Source: CAD feature listing. Evaluate the final solid. Frame: model axes, mm. A direction names the side the tool comes from. Round coordinates to 2 decimals unless told otherwise and drop trailing zeros. Loops run counter-clockwise (first coordinate to the right, second up) from the corner with the lowest first, then second, coordinate; pieces in that order, holes last. Notation, with made-up numbers: M -2,-27.75 L 26,-27.75 A35 cw 26,8.25 Z; hole C 86.5,7 d10. An arc over 180 degrees is marked long. Write each question's results on one line, items separated by ' | '. Start each with the question number.
1. Draft query along X for faces 1 (the flat face through (3, 14, 7)), 2 (the cylindrical face through (0.6, 27.43, 5.58)), 3 (the flat face through (101, 14, 1)), 4 (the flat face through (63.7, 25.2, 12)). Return one class per face: released by +X, released by -X, zero draft, split by the parting line, or undercut.
2. Ray query, line 1 (Y direction, x = 64, z = 8); line 2 (Y direction, x = 37, z = 9.75); line 3 (Z direction, x = 116, y = 22.25). Return the intervals inside material, ascending.
3. Section B-B on x = 58.5. Output: boundary loops of the cut face in (y, z).
4. Section C-C on x = 117. Output: boundary loops of the cut face in (y, z), and give its area (3 significant figures).
5. Set-up query: faces 5 (the flat face through (0, 14, 5)), 6 (the flat face through (64, 14, 2)), 7 (the flat face through (127, 14, 6)). Return all of +Z, -Z, +X, -X, +Y, -Y with unobstructed straight access to the full face (end or side cutting, diameter ignored); none if empty.
6. Section A-A on z = 9.75. Output: boundary loops of the cut face in (x, y).
7. Contact query for flat-ended pins moving along their axis: pin 1 Ø0.6 at (x, y) = (64.5, 14) entering from +Z; pin 2 Ø0.5 at (x, z) = (54, 11.5) entering from +Y; pin 3 Ø4 at (x, y) = (87.5, 18) entering from +Z. Output: stop coordinate, or through.
Autodesk Inventor part; units mm, degrees
ref_plane "Work Plane7" through (0, 0, 12) normal (0, 0, 1) x (1, 0, 0)
ref_plane "Work Plane6" through (0, 0, 12) normal (0, 0, 1) x (1, 0, 0)
ref_plane "Work Plane5" through (0, 0, 12) normal (0, 0, 1) x (1, 0, 0)
sketch "Sketch1" plane through (0, 0, 0) normal (0, 0, 1) x (1, 0, 0)
  line L0 (0, 0) -> (128, 0)
  line L1 (128, 0) -> (128, 28)
  line L2 (128, 28) -> (0, 28)
  line L3 (0, 28) -> (0, 0)
  dimension "d57" = 128
  dimension "d58" = 28
ref_plane "Work Plane7" through (0, 0, 12) normal (0, 0, 1) x (1, 0, 0)
sketch "Sketch2" plane through (0, 0, 12) normal (0, 0, 1) x (1, 0, 0)
  line L0 (3, 3) -> (85, 3)
  line L1 (85, 3) -> (85, 45)
  line L2 (85, 45) -> (3, 45)
  line L3 (3, 45) -> (3, 3)
  line L4 (88, 48) -> (0, 48)
  line L5 (88, 0) -> (88, 48)
  line L6 (0, 0) -> (88, 0)
  line L7 (0, 48) -> (0, 0)
  dimension "d4" = 3
  dimension "d5" = 3
  dimension "d6" = 3
  dimension "d7" = 3
ref_plane "Work Plane6" through (0, 0, 12) normal (0, 0, 1) x (1, 0, 0)
sketch "Sketch3" plane through (0, 0, 12) normal (0, 0, 1) x (1, 0, 0)
  line L0 (1.5, 46.5) -> (86.5, 46.5)
  line L1 (86.5, 46.5) -> (86.5, 1.5)
  line L2 (86.5, 1.5) -> (1.5, 1.5)
  line L3 (1.5, 1.5) -> (1.5, 46.5)
  line L4 (0, 0) -> (88, 0)
  line L5 (0, 48) -> (0, 0)
  line L6 (88, 0) -> (0, 0)
  line L7 (0, 0) -> (0, 48)
  line L8 (0, 48) -> (88, 48)
  line L9 (88, 48) -> (88, 0)
  dimension "d10" = 1.5
  dimension "d11" = 1.5
  dimension "d12" = 1.5
  dimension "d13" = 1.5
ref_plane "Work Plane5" through (0, 0, 12) normal (0, 0, 1) x (1, 0, 0)
sketch "Sketch4" plane through (0, 0, 12) normal (0, 0, 1) x (1, 0, 0)
  circle A0 centre (5.5, 24) radius 1
  circle A1 centre (82.5, 24) radius 1
  line L0 (3, 45) -> (85, 45)
  line L1 (3, 3) -> (3, 45)
  line L2 (3, 25.5) -> (5.5, 25.5)
  line L3 (5.5, 25.5) -> (5.5, 22.5)
  line L4 (5.5, 22.5) -> (3, 22.5)
  line L5 (3, 22.5) -> (3, 25.5)
  circle A2 centre (5.5, 24) radius 1.5
  line L6 (85, 45) -> (85, 3)
  line L7 (85, 22.5) -> (82.5, 22.5)
  line L8 (82.5, 22.5) -> (82.5, 25.5)
  line L9 (82.5, 25.5) -> (85, 25.5)
  line L10 (85, 25.5) -> (85, 22.5)
  circle A3 centre (82.5, 24) radius 1.5
  point P0 (0, 0)
  dimension "d17" = 2
  dimension "d18" = 2
  dimension "d19" = 21
  dimension "d20" = 21
  dimension "d21" = 2.5
  dimension "d22" = 3
  dimension "d23" = 1.5
  dimension "d24" = 2.5
  dimension "d25" = 2.5
  dimension "d26" = 3
  dimension "d27" = 1.5
ref_plane "Work Plane4" through (0, 0, 12) normal (0, 0, 1) x (1, 0, 0)
sketch "Sketch5" plane through (0, 0, 12) normal (0, 0, 1) x (1, 0, 0)
  circle A0 centre (5.5, 24) radius 1
  circle A1 centre (82.5, 24) radius 1
  line L0 (3, 25.5) -> (3, 22.5)
  line L1 (3, 22.5) -> (5.5, 22.5)
  line L2 (82.5, 22.5) -> (85, 22.5)
  line L3 (85, 22.5) -> (85, 25.5)
  point P0 (0, 0)
  dimension "d30" = 2
  dimension "d31" = 2
  dimension "d32" = 2.5
  dimension "d33" = 1.5
  dimension "d34" = 1.5
  dimension "d35" = 2.5
ref_plane "Work Plane1" through (0, 0, 3) normal (0, 0, 1) x (1, 0, 0)
sketch "Sketch6" plane through (0, 0, 3) normal (0, 0, 1) x (1, 0, 0)
  line L0 (35, 45) -> (53, 45)
  line L1 (53, 45) -> (53, 9)
  line L2 (53, 9) -> (35, 9)
  line L3 (35, 9) -> (35, 45)
  line L4 (3, 45) -> (85, 45)
  line L5 (3, 3) -> (3, 45)
  point P0 (0, 0)
  point P1 (3, 25.5)
  dimension "d38" = 18
  dimension "d39" = 36
  dimension "d40" = 0
  dimension "d41" = 32
  dimension "d50" = 82
ref_plane "Work Plane2" through (0, 48, 11) normal (0, 1, 0) x (1, 0, 0)
sketch "Sketch7" plane through (0, 48, 11) normal (0, 1, 0) x (1, 0, 0)
  line L0 (48.5, 4.8) -> (40.5, 4.8)
  line L1 (40.5, 4.8) -> (40.5, 8)
  line L2 (40.5, 8) -> (48.5, 8)
  line L3 (48.5, 8) -> (48.5, 4.8)
  line L4 (88, 11) -> (0, 11)
  line L5 (86, 11) -> (86, 0)
  dimension "d44" = 8
  dimension "d45" = 3.2
  dimension "d46" = 3
  dimension "d47" = 37.5
ref_plane "Work Plane3" through (0, 48, 11) normal (0, 1, 0) x (1, 0, 0)
sketch "Sketch8" plane through (0, 48, 11) normal (0, 1, 0) x (1, 0, 0)
  line L0 (50.5, 9.5) -> (38.5, 9.5)
  line L1 (38.5, 9.5) -> (38.5, 3.3)
  line L2 (38.5, 3.3) -> (50.5, 3.3)
  line L3 (50.5, 3.3) -> (50.5, 9.5)
  line L4 (48.5, 8) -> (48.5, 4.8)
  line L5 (40.5, 4.8) -> (40.5, 8)
  line L6 (48.5, 4.8) -> (40.5, 4.8)
  line L7 (40.5, 8) -> (48.5, 8)
  point P0 (0, 11)
  dimension "d51" = 2
  dimension "d52" = 2
  dimension "d53" = 1.5
  dimension "d54" = 1.5
extrude "Extrusion9" add sketch "Sketch1" along normal blind 11
sketch "Sketch9" plane through (0, 0, 11) normal (0, 0, 1) x (1, 0, 0)
  line L0 (3, 3) -> (125, 3)
  line L1 (125, 3) -> (125, 25)
  line L2 (125, 25) -> (3, 25)
  line L3 (3, 25) -> (3, 3)
  line L4 (0, 0) -> (128, 0)
  line L5 (0, 28) -> (0, 0)
  dimension "d61" = 122
  dimension "d62" = 22
  dimension "d63" = 3
  dimension "d64" = 3
extrude "Extrusion10" cut sketch "Sketch9" against normal blind 9
fillet "Fillet2" radius 2 4 edges at (128, 0, 5.5) (0, 28, 5.5) (0, 0, 5.5) (128, 28, 5.5)
sketch "Sketch10" plane through (0, 0, 11) normal (0, 0, 1) x (1, 0, 0)
  line L0 (3, 3) -> (3, 25)
  line L1 (125, 25) -> (125, 3)
  line L2 (3, 25) -> (125, 25)
  line L3 (125, 25) -> (125, 3)
  line L4 (125, 3) -> (3, 3)
  line L5 (3, 3) -> (3, 25)
  line L6 (1.5, 26.5) -> (126.5, 26.5)
  line L7 (126.5, 26.5) -> (126.5, 1.5)
  line L8 (126.5, 1.5) -> (1.5, 1.5)
  line L9 (1.5, 1.5) -> (1.5, 26.5)
  point P0 (0, 0)
  dimension "d69" = 1.5
  dimension "d70" = 1.5
  dimension "d71" = 1.5
  dimension "d72" = 1.5
extrude "Extrusion11" add sketch "Sketch10" along normal blind 1
sketch "Sketch11" plane through (0, 0, 2) normal (0, 0, 1) x (1, 0, 0)
  line L0 (125, 5.15) -> (77, 5.15)
  line L1 (77, 5.15) -> (77, 22.85)
  line L2 (77, 22.85) -> (125, 22.85)
  line L3 (125, 22.85) -> (125, 5.15)
  line L4 (125, 25) -> (125, 3)
  line L5 (3, 25) -> (125, 25)
  point P0 (0, 0)
  dimension "d75" = 48
  dimension "d76" = 17.7
  dimension "d77" = 0
  dimension "d78" = 2.15
extrude "Extrusion12" cut sketch "Sketch11" against normal blind 1
sketch "Sketch13" plane through (128, 2, 0) normal (1, 0, 0) x (0, 0, -1)
  line L0 (-2, 7) -> (-6, 7)
  line L1 (-6, 7) -> (-6, 17)
  line L2 (-6, 17) -> (-2, 17)
  line L3 (-2, 17) -> (-2, 7)
  line L4 (-11, -2) -> (0, -2)
  line L5 (0, 0) -> (0, 24)
  dimension "d81" = 4
  dimension "d82" = 10
  dimension "d83" = 9
  dimension "d84" = 2
extrude "Extrusion13" cut sketch "Sketch13" against normal blind 3
sketch "Sketch14" plane through (0, 0, 2) normal (0, 0, 1) x (1, 0, 0)
  circle A0 centre (64, 14) radius 1
  circle A1 centre (64, 14) radius 2
  line L0 (3, 25) -> (125, 25)
  line L1 (3, 3) -> (3, 25)
  point P0 (0, 0)
  dimension "d87" = 2
  dimension "d88" = 4
  dimension "d89" = 11
  dimension "d90" = 61
extrude "Extrusion14" add sketch "Sketch14" along normal blind 10
properties part number "Base Wide"
Taken from the geometry:
1) face 1: undercut | face 2: released by -X | face 3: undercut | face 4: zero draft
2) line 1: 0 to 3, 12 to 13, 15 to 16, 25 to 28 | line 2: 0 to 3, 25 to 28 | line 3: 0 to 1
3) outline: M 0,0 L 28,0 L 28,11 L 26.5,11 L 26.5,12 L 25,12 L 25,2 L 3,2 L 3,12 L 1.5,12 L 1.5,11 L 0,11 Z
4) outline: M 0,0 L 28,0 L 28,11 L 26.5,11 L 26.5,12 L 25,12 L 25,2 L 22.85,2 L 22.85,1 L 5.15,1 L 5.15,2 L 3,2 L 3,12 L 1.5,12 L 1.5,11 L 0,11 Z | area: 95.3 mm^2
5) face 5: +Z, -Z, -X, +Y, -Y | face 6: +Z | face 7: +X
6) outline: M 0,2 A2 ccw 2,0 L 126,0 A2 ccw 128,2 L 128,26 A2 ccw 126,28 L 2,28 A2 ccw 0,26 Z; C 64,14 d4; hole M 3,3 L 125,3 L 125,25 L 3,25 Z; hole C 64,14 d2
7) pin 1: z = 2 | pin 2: y = 26.5 | pin 3: z = 1
